```python
from build123d import *

# Parameters (mm, degrees)
SKETCH1_R             = 3.125
BOSS_EXTRUDE1_DEPTH   = 3
BOSS_EXTRUDE1_2_DEPTH = 3
BOSS_EXTRUDE1_3_DEPTH = 3
BOSS_EXTRUDE1_4_DEPTH = 3
BOSS_EXTRUDE2_DEPTH   = 1


with BuildPart() as part:
    # Sketch1 → Boss-Extrude1 (new body)
    with BuildSketch(Plane(origin=(0, 0, 0), x_dir=(1, 0, 0), z_dir=(0, 1, 0))):
        with Locations(Location((20, -15, 0), (0, 0, 270))):
            Circle(SKETCH1_R)
    extrude(amount=BOSS_EXTRUDE1_DEPTH)



with BuildPart() as body_2:
    # Sketch1 → Boss-Extrude1 2 (new body)
    with BuildSketch(Plane(origin=(0, 0, 0), x_dir=(1, 0, 0), z_dir=(0, 1, 0))):
        with Locations(Location((-13.25542136, 9.94156602, 0), (0, 0, 270))):
            Circle(SKETCH1_R)
    extrude(amount=BOSS_EXTRUDE1_2_DEPTH)


with BuildPart() as body_3:
    # Sketch1 → Boss-Extrude1 3 (new body)
    with BuildSketch(Plane(origin=(0, 0, 0), x_dir=(1, 0, 0), z_dir=(0, 1, 0))):
        with BuildLine():
            Line((-6.119805779, -13.831616038), (16.156155048, -23.687626603))
            ThreePointArc((16.156155048, -23.687626603), (27.344292117, -21.025891909), (27.769542612, -9.533354996))
            Line((27.769542612, -9.533354996), (15.950313209, 7.264883492))
            ThreePointArc((15.950313209, 7.264883492), (12.8913772, 10.324262075), (8.979166667, 12.17128551))
            ThreePointArc((8.979166667, 12.17128551), (6.819498906, 13.500372575), (4.468133972, 14.44996207))
            Line((4.468133972, 14.44996207), (-10.436297143, 19.05862434))
            ThreePointArc((-10.436297143, 19.05862434), (-20.352140796, 16.321596348), (-22.022063001, 6.171392537))
            Line((-22.022063001, 6.171392537), (-17.222949988, -4.987803231))
            ThreePointArc((-17.222949988, -4.987803231), (-13.919097451, -9.518328239), (-8.979166667, -12.17128551))
            ThreePointArc((-8.979166667, -12.17128551), (-7.594992863, -13.079820657), (-6.119805779, -13.831616038))
        make_face()
        with BuildLine():
            Line((-5.310575263, -12.002642017), (16.965385564, -21.858652581))
            ThreePointArc((16.965385564, -21.858652581), (25.798125356, -19.757283086), (26.133849431, -10.684227629))
            Line((26.133849431, -10.684227629), (14.314620027, 6.114010859))
            ThreePointArc((14.314620027, 6.114010859), (11.588405557, 8.793657895), (8.090277778, 10.335038968))
            ThreePointArc((8.090277778, 10.335038968), (6.084437075, 11.62949915), (3.877306339, 12.539223283))
            Line((3.877306339, 12.539223283), (-11.027124776, 17.147885554))
            ThreePointArc((-11.027124776, 17.147885554), (-18.864821465, 14.984479597), (-20.184763993, 6.961539583))
            Line((-20.184763993, 6.961539583), (-15.38565098, -4.197656185))
            ThreePointArc((-15.38565098, -4.197656185), (-12.464970786, -8.130524254), (-8.090277778, -10.335038968))
            ThreePointArc((-8.090277778, -10.335038968), (-6.752106378, -11.254984872), (-5.310575263, -12.002642017))
        make_face(mode=Mode.SUBTRACT)
    extrude(amount=BOSS_EXTRUDE1_3_DEPTH)


with BuildPart() as body_4:
    # Sketch1 → Boss-Extrude1 4 (new body)
    with BuildSketch(Plane(origin=(0, 0, 0), x_dir=(1, 0, 0), z_dir=(0, 1, 0))):
        with BuildLine():
            ThreePointArc((-5.868055556, -5.619746346), (0, -8.125), (5.868055556, -5.619746346))
            ThreePointArc((5.868055556, -5.619746346), (11.25, 0), (5.868055556, 5.619746346))
            ThreePointArc((5.868055556, 5.619746346), (0, 8.125), (-5.868055556, 5.619746346))
            ThreePointArc((-5.868055556, 5.619746346), (-11.25, 0), (-5.868055556, -5.619746346))
        make_face()
    extrude(amount=BOSS_EXTRUDE1_4_DEPTH)


with BuildPart() as part_1:
    add(part.part)

    add(body_2.part)  # Boss-Extrude2 merges body 2

    add(body_3.part)  # Boss-Extrude2 merges body 3

    add(body_4.part)  # Boss-Extrude2 merges body 4
    # Sketch2 → Boss-Extrude2 (add)
    with BuildSketch(Plane.XZ):
        with BuildLine():
            Line((-17.222949988, 4.987803231), (-22.022063001, -6.171392537))
            ThreePointArc((-22.022063001, -6.171392537), (-20.352140796, -16.321596348), (-10.436297143, -19.05862434))
            Line((-10.436297143, -19.05862434), (4.468133972, -14.44996207))
            ThreePointArc((4.468133972, -14.44996207), (6.819498906, -13.500372575), (8.979166667, -12.17128551))
            ThreePointArc((8.979166667, -12.17128551), (12.8913772, -10.324262075), (15.950313209, -7.264883492))
            Line((15.950313209, -7.264883492), (27.769542612, 9.533354996))
            ThreePointArc((27.769542612, 9.533354996), (27.344292117, 21.025891909), (16.156155048, 23.687626603))
            Line((16.156155048, 23.687626603), (-6.119805779, 13.831616038))
            ThreePointArc((-6.119805779, 13.831616038), (-7.594992863, 13.079820657), (-8.979166667, 12.17128551))
            ThreePointArc((-8.979166667, 12.17128551), (-13.919097451, 9.518328239), (-17.222949988, 4.987803231))
        make_face()
    extrude(amount=BOSS_EXTRUDE2_DEPTH)


solid = part_1.part
```
Geometry check sheet. Reference: the model listing, model coordinates, mm. A direction names the side the tool comes from. Give positions to 0.01 mm unless a question says otherwise; leave off trailing zeros. Order: outer loops, then holes, each group sorted by start corner. A loop starts at its lowest first (then second) coordinate and runs counter-clockwise, first axis right, second up. Notation, with made-up numbers: (-21.75, 41.25) - (21.25, 41.25) arc R24 ccw to (21.25, 66.25) - close; hole circle Ø1 at (87, 54.25). An arc over 180 degrees is marked (long way). Write item = value, one per line. Start each with the question number.
1) Section check B-B (x = 10). Enter the section's corners in (y, z), then the cut area to 3 significant figures.
2) Gauge pin test, flat ends, axial feed: pin 1 Ø1 at (x, y) = (13, 0) entering from -Z; pin 2 Ø2 at (y, z) = (-0.5, 7) entering from -X; pin 3 Ø1 at (x, y) = (-10, 2) entering from +Z. Record the tip position at first contact, or that the pin passes through.
3) Section check A-A (y = 1.6). Enter the section's corners in (x, z) (3 decimals), then the cut area to 3 significant figures.
4) Access from +Z, -Z, +X, -X, +Y, -Y to the whole of each face (thin tool, end or side, straight path). Record for faces 1 (the flat face through (20, 3, 15)), 2 (the cylindrical face through (11.633, 1.479, -8.763)).
5) Section check D-D (x = 25). Enter the section's corners in (y, z).
6) Scan lines: L1, parallel to X at y = 0.2, z = 15 (3 decimals); L2, parallel to X at y = 1.55, z = -4; L3, parallel to Z at x = -6.5, y = 2. Record each from-to range of solid material in increasing order.
7) Section check C-C (z = 0). Enter the section's corners in (x, y), then the cut area to 3 significant figures.
Geometry check:
q1.outline = (-1, -11.84) - (3, -11.84) - (3, -9.68) - (0, -9.68) - (0, -3.54) - (3, -3.54) - (3, 3.54) - (0, 3.54) - (0, 18.78) - (3, 18.78) - (3, 20.96) - (-1, 20.96) - close
q1.area = 67.1 mm2
q2.pin_1 = -10.59
q2.pin_2 = -16.73
q2.pin_3 = 12.02
q3.outline = (-22.022, -6.171) arc R9.543 ccw to (-10.436, -19.059) - (4.468, -14.45) arc R15.125 ccw to (8.979, -12.171) arc R12.625 ccw to (15.95, -7.265) - (27.77, 9.533) arc R9.5 ccw to (16.156, 23.688) - (-6.12, 13.832) arc R15.125 ccw to (-8.979, 12.171) arc R12.625 ccw to (-17.223, 4.988) - close; circle Ø6.25 at (-13.255, -9.942); (-5.868, -5.62) arc R8.125 ccw to (5.868, -5.62) arc R5.625 ccw to (5.868, 5.62) arc R8.125 ccw to (-5.868, 5.62) arc R5.625 ccw to start; circle Ø6.25 at (20, 15); hole (-20.185, -6.962) arc R7.543 ccw to (-11.027, -17.148) - (3.877, -12.539) arc R13.125 ccw to (8.09, -10.335) arc R10.625 ccw to (14.315, -6.114) - (26.134, 10.684) arc R7.5 ccw to (16.965, 21.859) - (-5.311, 12.003) arc R13.125 ccw to (-8.09, 10.335) arc R10.625 ccw to (-15.386, 4.198) - close
q3.area = 610 mm2
q4.face_1 = +Z, -Z, +X, -X, +Y
q4.face_2 = +Y
q5.outline = (-1, 5.6) - (3, 5.6) - (3, 9.07) - (0, 9.07) - (0, 20.59) - (3, 20.59) - (3, 23.08) - (-1, 23.08) - close
q6.L1 = -3.479 to 1.464, 16.875 to 23.125, 27.5 to 29.5
q6.L2 = -21.09 to -18.91, -9.58 to 9.58, 15.8 to 18.25
q6.L3 = -17.84 to -15.75, -5.56 to 5.56, 11.4 to 13.66
q7.outline = (-19.37, -1) - (21.06, -1) - (21.06, 3) - (18.62, 3) - (18.62, 0) - (11.25, 0) - (11.25, 3) - (-11.25, 3) - (-11.25, 0) - (-17.19, 0) - (-17.19, 3) - (-19.37, 3) - close
q7.area = 122 mm2
